The listing builds one solid part. Answer for the finished solid, in the listing's coordinates (mm). Give positions to 0.01 mm unless a question says otherwise; leave off trailing zeros. Write each loop counter-clockwise with the first axis right and the second up, starting at its lowest first coordinate (ties: lowest second). Pieces come first, ordered by that corner, then holes. Notation, with made-up numbers: M 67.25,-5 L 108.25,-5 A19 ccw 108.25,10 Z; hole C 5,-4 d8. An arc over 180 degrees is marked long. Return JSON: item names as keys, results as strings.
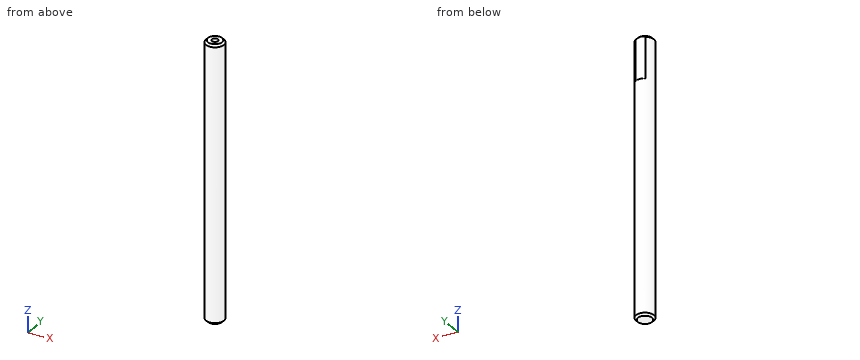
from build123d import *

# Parameters (mm, degrees)
IZIM1_R                     = 3.175
Y_KSEKLIK_EKSTR_ZYON1_DEPTH = 96.6
IZIM3_R                     = 1.1
KES_EKSTR_ZYON2_DEPTH       = 25
PAH1_SIZE                   = 0.7
PAH2_SIZE                   = 0.7
CORTE_EXTRUS_O1_START       = -15
CORTE_EXTRUS_O1_DEPTH       = 15


with BuildPart() as part:
    # Çizim1 → Yükseklik-Ekstrüzyon1 (new body)
    with BuildSketch(Plane.XY):
        with Locations(Location((0, 0, 0), (0, 0, 180))):
            Circle(IZIM1_R)
    extrude(amount=Y_KSEKLIK_EKSTR_ZYON1_DEPTH)

    # Çizim3 → Kes-Ekstrüzyon2 (cut)
    with BuildSketch(Plane.XY.offset(96.6)):
        Circle(IZIM3_R)
    extrude(amount=-KES_EKSTR_ZYON2_DEPTH, mode=Mode.SUBTRACT)

    # Pah1
    pah1_edges = [part.edges().sort_by_distance(p)[0] for p in [
        (3.175, 0, 96.6),
    ]]
    chamfer(pah1_edges, length=PAH1_SIZE)

    # Pah2
    pah2_edges = [part.edges().sort_by_distance(p)[0] for p in [
        (3.175, 0, 0),
    ]]
    chamfer(pah2_edges, length=PAH2_SIZE)

    # Esboço1 → Corte-extrusão1 (cut)
    with BuildSketch(Plane.XY.offset(96.6).offset(CORTE_EXTRUS_O1_START)):
        with BuildLine():
            Line((-1.78605711, 2.625), (1.78605711, 2.625))
            ThreePointArc((1.78605711, 2.625), (0, 3.175), (-1.78605711, 2.625))
        make_face()
    extrude(amount=CORTE_EXTRUS_O1_DEPTH, mode=Mode.SUBTRACT)


solid = part.part
Item 1: A cutting plane is placed at D-D, the plane z = 27.5. Write down the section's boundary in (x, y) (3 decimals).
Geometry results:
{"outline": "C 0,0 d6.35"}
Item 2: A cutting plane is placed at C-C, the plane z = 79.5. Write down the section's boundary in (x, y) (3 decimals), plus the area to 3 significant figures.
Geometry results:
{"outline": "C 0,0 d6.35; hole C 0,0 d2.2", "area": "27.9 mm2"}
Item 3: A cutting plane is placed at A-A, the plane y = 0. Write down the section's boundary in (x, z) (3 decimals).
Geometry results:
{"outline": "M -3.175,0.7 L -2.475,0 L 2.475,0 L 3.175,0.7 L 3.175,95.9 L 2.475,96.6 L 1.1,96.6 L 1.1,71.6 L -1.1,71.6 L -1.1,96.6 L -2.475,96.6 L -3.175,95.9 Z"}
Item 4: A cutting plane is placed at B-B, the plane x = 0. Write down the section's boundary in (y, z) (3 decimals).
Geometry results:
{"outline": "M -3.175,0.7 L -2.475,0 L 2.475,0 L 3.175,0.7 L 3.175,81.6 L 2.625,81.6 L 2.625,96.45 L 2.475,96.6 L 1.1,96.6 L 1.1,71.6 L -1.1,71.6 L -1.1,96.6 L -2.475,96.6 L -3.175,95.9 Z"}
Item 5: Given pin 1 Ø1.5 at (x, z) = (1.5, 25) entering from -Y; pin 2 Ø3 at (y, z) = (2.5, 81.5) entering from +X; pin 3 Ø3 at (y, z) = (-1, 60) entering from +X (3 decimals); pin 4 Ø1.1 at (x, y) = (0, 0.5) entering from +Z, each flat-ended and moving along its own axis, determine where each tip first touches the part or whether it passes through.
Geometry results:
{"pin 1": "stops at y = -3.09", "pin 2": "stops at x = 3.01", "pin 3": "stops at x = 3.175", "pin 4": "stops at z = 71.6"}
Item 6: Find the intervals of material crossed by line 1 (Y direction, x = 0, z = 82.5) (3 decimals); line 2 (Y direction, x = 0, z = 77.75) (3 decimals); line 3 (Z direction, x = -0.75, y = -0.5), in increasing order.
Geometry results:
{"line 1": "y = -3.175 to -1.1, 1.1 to 2.625", "line 2": "y = -3.175 to -1.1, 1.1 to 3.175", "line 3": "z = 0 to 71.6"}
